from build123d import *

# Parameters (mm, degrees)
BOSS_EXTRUDE1_DEPTH = 5
SKETCH2_R           = 5
SKETCH2_R_2         = 2.5
CUT_EXTRUDE1_DEPTH  = 6
SKETCH4_W           = 20
SKETCH4_H           = 11
CUT_EXTRUDE3_DEPTH  = 10
BOSS_EXTRUDE3_DEPTH = 6
SKETCH7_R           = 1.25
SKETCH7_R_2         = 12
CUT_EXTRUDE4_DEPTH  = 6
SKETCH9_W           = 20
SKETCH9_H           = 180
CUT_EXTRUDE5_DEPTH  = 6
FILLET1_R           = 5


with BuildPart() as part:
    # Sketch1 → Boss-Extrude1 (new body)
    with BuildSketch(Plane(origin=(0, 0, 0), x_dir=(1, 0, 0), z_dir=(0, 1, 0))):
        Polygon((0, 0), (30, 0), (30, 12), (70, 12), (70, 0), (100, 0), (100, 300), (0, 300), align=None)
    extrude(amount=BOSS_EXTRUDE1_DEPTH)

    # Sketch2 → Cut-Extrude1 (cut)
    with BuildSketch(Plane(origin=(0, 5, 0), x_dir=(1, 0, 0), z_dir=(0, 1, 0))):
        with Locations(Location((72, 27, 0), (0, 0, 270))):
            Circle(SKETCH2_R)
        with Locations(Location((88.403124702, 19, 0), (0, 0, 270))):
            Circle(SKETCH2_R_2)
        with Locations(Location((55.596875298, 35, 0), (0, 0, 270))):
            Circle(SKETCH2_R_2)
    extrude(amount=-CUT_EXTRUDE1_DEPTH, mode=Mode.SUBTRACT)

    # Sketch4 → Cut-Extrude3 (cut)
    with BuildSketch(Plane(origin=(0, 5, 0), x_dir=(1, 0, 0), z_dir=(0, 1, 0))):
        with Locations((40, 294.5)):
            Rectangle(SKETCH4_W, SKETCH4_H)
    extrude(amount=-CUT_EXTRUDE3_DEPTH, mode=Mode.SUBTRACT)

    # Sketch6 → Boss-Extrude3 (add)
    with BuildSketch(Plane(origin=(0, 5, 0), x_dir=(1, 0, 0), z_dir=(0, 1, 0))):
        Polygon((100, 0), (100, 150), (140, 120), (140, 20), align=None)
    extrude(amount=-BOSS_EXTRUDE3_DEPTH)

    # Sketch7 → Cut-Extrude4 (cut)
    with BuildSketch(Plane(origin=(0, 5, 0), x_dir=(1, 0, 0), z_dir=(0, 1, 0))):
        with Locations(Location((130.5, 60.5, 0), (0, 0, 270))):
            Circle(SKETCH7_R)
        with Locations(Location((99.5, 60.5, 0), (0, 0, 270))):
            Circle(SKETCH7_R)
        with Locations(Location((99.5, 29.5, 0), (0, 0, 270))):
            Circle(SKETCH7_R)
        with Locations(Location((130.5, 29.5, 0), (0, 0, 270))):
            Circle(SKETCH7_R)
        with Locations(Location((115, 45, 0), (0, 0, 270))):
            Circle(SKETCH7_R_2)
    extrude(amount=-CUT_EXTRUDE4_DEPTH, mode=Mode.SUBTRACT)

    # Sketch9 → Cut-Extrude5 (cut)
    with BuildSketch(Plane(origin=(0, 5, 0), x_dir=(1, 0, 0), z_dir=(0, 1, 0))):
        Polygon((100, 300), (90, 300), (100, 150), align=None)
        with Locations((50, 150)):
            Rectangle(SKETCH9_W, SKETCH9_H)
    extrude(amount=-CUT_EXTRUDE5_DEPTH, mode=Mode.SUBTRACT)

    # Fillet1
    fillet1_edges = [part.edges().sort_by_distance(p)[0] for p in [
        (60, 2.5, -240),
        (60, 2.5, -60),
        (40, 2.5, -60),
        (40, 2.5, -240),
    ]]
    fillet(fillet1_edges, radius=FILLET1_R)


solid = part.part
Check sheet for the modelled part. Datum: model origin and axes. Units: mm. A direction names the side the tool comes from. Give positions to 0.01 mm unless a question says otherwise; leave off trailing zeros. Loops run counter-clockwise (first coordinate to the right, second up) from the corner with the lowest first, then second, coordinate; pieces in that order, holes last. Notation, with made-up numbers: M 50,27.5 L 70,27.5 A14 cw 70,47.5 Z; hole C 79,82 d9. An arc over 180 degrees is marked long. Use a Markdown table: item, result. Add a question column.
Q1. Sectioned sample at A-A, the plane z = -81. Record the cut outline in (x, y).
Q2. Go/stop test with flat-tipped pins: pin 1 (1 mm diameter, centred on x = 16.5, z = -252.5, fed in from -Y); pin 2 (1.5 mm diameter, centred on x = 51.5, y = 1.5, fed in from +Z); pin 3 (1.5 mm diameter, centred on x = 44, y = 2.5, fed in from -Z). Record where each tip stops, or that it passes through.
Q3. Tool access check on faces 4 (the flat face through (50, 3, -294)), 5 (the flat face through (70, 2, -6)), 6 (the cylindrical face through (58, 2, -61)). Record the directions out of +Z, -Z, +X, -X, +Y, -Y that give a thin tool (end or side, any length) a straight path to the whole face; none if there is none.
Q4. Mould release check, pull along Z, two halves, no side actions. Record for faces 1 (the flat face through (38, 0, -152)), 2 (the flat face through (50, 2, -12)), 3 (the flat face through (50, 3, -240)): pulls with the +Z half, pulls with the -Z half, needs draft (parallel to the pull), parting line crosses it, or undercut.
Q5. Scan lines: line 1 along X through (y, z) = (2.05, -29.5); line 2 along Y through (x, z) = (81.5, -285.5); line 3 along X through (y, z) = (2.55, -44.5). Record each from-to range of solid material in increasing order. Write a range as [from, to].
Q6. Sectioned sample at C-C, the plane y = 1.3. Give the number of separate pieces and of enclosed holes in the cut face, then the cut area to 3 significant figures.
Q7. Sectioned sample at D-D, the plane z = -45. Record the cut outline in (x, y).
Q8. Sectioned sample at B-B, the plane x = 115. Record the cut outline in (y, z), then the cut area to 4 significant figures.
Verdict:
| question | item | result |
|---|---|---|
| 1 | outline | M 0,0 L 40,0 L 40,5 L 0,5 Z; M 60,0 L 100,0 L 100,-1 L 140,-1 L 140,5 L 60,5 Z |
| 2 | pin 1 | y = 0 |
| 2 | pin 2 | z = -12 |
| 2 | pin 3 | z = -289 |
| 3 | face 4 | -Z, +Y, -Y |
| 3 | face 5 | +Z, +Y, -Y |
| 3 | face 6 | +Y, -Y |
| 4 | face 1 | needs draft |
| 4 | face 2 | pulls with the +Z half |
| 4 | face 3 | undercut |
| 5 | line 1 | [0, 67.67], [76.33, 98.25], [100.75, 129.25], [131.75, 140] |
| 5 | line 2 | [0, 5] |
| 5 | line 3 | [0, 103.01], [126.99, 140] |
| 6 | separate pieces | 1 |
| 6 | enclosed holes | 9 |
| 6 | area | 29,400 mm^2 |
| 7 | outline | M 0,0 L 100,0 L 100,-1 L 103,-1 L 103,5 L 0,5 Z; M 127,-1 L 140,-1 L 140,5 L 127,5 Z |
| 8 | outline | M -1,-138.75 L 5,-138.75 L 5,-57 L -1,-57 Z; M -1,-33 L 5,-33 L 5,-7.5 L -1,-7.5 Z |
| 8 | area | 643.5 mm^2 |
